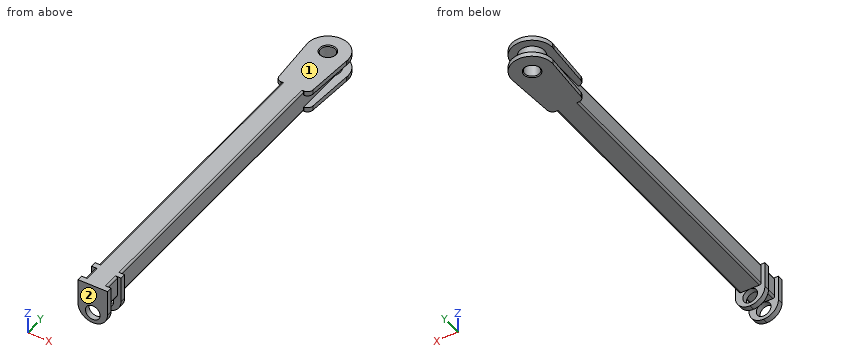
```python
from build123d import *

# Parameters (mm, degrees)
F0_W      = 120
F0_H      = 120
F0_W_2    = 100
F0_H_2    = 100
F1_DEPTH  = 1000
F2_R      = 67.5
F3_DEPTH  = 120
F4_R      = 40
F5_DEPTH  = 120
F7_DEPTH  = 25
F9_DEPTH  = 25
F10_R     = 40
F11_DEPTH = 160
F12_W     = 30
F12_H     = 220
F13_DEPTH = 140
F14_W     = 30
F14_H     = 220
F15_DEPTH = 20
F16_W     = 30
F16_H     = 220
F17_DEPTH = 140
F18_W     = 30
F18_H     = 220
F19_DEPTH = 20
F20_R     = 40
F21_DEPTH = 145
F22_R     = 10
F23_R     = 79.99999
F24_R     = 30
F25_SIZE  = 5


# Not quite as in the source:
# - a fillet or chamfer is up to 0.001 mm smaller than in the source, because OpenCascade refuses the exact size


with BuildPart() as f1:
    # F0 (on Front) → F1 (new body, symmetric)
    with BuildSketch(Plane.XZ):
        Rectangle(F0_W, F0_H)
        Rectangle(F0_W_2, F0_H_2, mode=Mode.SUBTRACT)
    extrude(amount=F1_DEPTH, both=True)

    # F2 (on face) → F3 (join)
    with BuildSketch(Plane.XY.offset(60)):
        with Locations((0, 1000)):
            Circle(F2_R)
    extrude(amount=-F3_DEPTH)

    # F4 (on face) → F5 (cut)
    with BuildSketch(Plane.XY.offset(60)):
        with Locations((0, 1000)):
            Circle(F4_R)
    extrude(amount=-F5_DEPTH, mode=Mode.SUBTRACT)

    # F6 (on face) → F7 (join)
    with BuildSketch(Plane.XY.offset(60)):
        with BuildLine():
            Line((109.0265486726, 985.3982300885), (110, 1000))
            ThreePointArc((110, 1000), (0, 1110), (-110, 1000))
            Line((-110, 1000), (-109.0265486726, 985.3982300885))
            ThreePointArc((-109.0265486726, 985.3982300885), (0, 890), (109.0265486726, 985.3982300885))
        make_face()
        with BuildLine():
            ThreePointArc((109.0265486726, 985.3982300885), (109.7563673642, 992.6829088424), (110, 1000))
            Line((110, 1000), (109.0265486726, 985.3982300885))
        make_face()
        with BuildLine():
            Line((-109.0265486726, 985.3982300885), (-110, 1000))
            ThreePointArc((-110, 1000), (-109.7563673642, 992.6829088424), (-109.0265486726, 985.3982300885))
        make_face()
        with BuildLine():
            Line((90, 700), (109.0265486726, 985.3982300885))
            ThreePointArc((109.0265486726, 985.3982300885), (0, 890), (-109.0265486726, 985.3982300885))
            Line((-109.0265486726, 985.3982300885), (-90, 700))
            Line((-90, 700), (90, 700))
        make_face()
    extrude(amount=-F7_DEPTH)

    # F8 (on face) → F9 (join)
    with BuildSketch(Plane(origin=(0, 0, -60), x_dir=(1, 0, 0), z_dir=(0, 0, -1))):
        with BuildLine():
            Line((109.0265486726, -985.3982300885), (110, -1000))
            ThreePointArc((110, -1000), (109.7563673642, -992.6829088424), (109.0265486726, -985.3982300885))
        make_face()
        with BuildLine():
            ThreePointArc((-109.7502513746, -992.5917395282), (-3.706234531, -1109.9375451136), (110, -1000))
            Line((110, -1000), (109.0265486726, -985.3982300885))
            ThreePointArc((109.0265486726, -985.3982300885), (-3.6149109138, -890.0594141407), (-109.7502513746, -992.5917395282))
        make_face()
        with BuildLine():
            ThreePointArc((-109.7502513746, -992.5917395282), (-3.6149109138, -890.0594141407), (109.0265486726, -985.3982300885))
            Line((109.0265486726, -985.3982300885), (90, -700))
            Line((90, -700), (-90, -700))
            Line((-90, -700), (-109.7502513746, -992.5917395282))
        make_face()
    extrude(amount=-F9_DEPTH)

    # F10 (on face) → F11 (cut)
    with BuildSketch(Plane(origin=(0, 0, -60), x_dir=(1, 0, 0), z_dir=(0, 0, -1))):
        with Locations((0, -1000)):
            Circle(F10_R)
    extrude(amount=-F11_DEPTH, mode=Mode.SUBTRACT)

    # F12 (on face) → F13 (join)
    with BuildSketch(Plane.YZ.offset(60)):
        with Locations((-870, -50)):
            Rectangle(F12_W, F12_H)
    extrude(amount=-F13_DEPTH)

    # F14 (on face) → F15 (join)
    with BuildSketch(Plane.YZ.offset(60)):
        with Locations((-870, -50)):
            Rectangle(F14_W, F14_H)
    extrude(amount=F15_DEPTH)

    # F16 (on face) → F17 (join)
    with BuildSketch(Plane.YZ.offset(60)):
        with Locations((-985, -50)):
            Rectangle(F16_W, F16_H)
    extrude(amount=-F17_DEPTH)

    # F18 (on face) → F19 (join)
    with BuildSketch(Plane.YZ.offset(60)):
        with Locations((-985, -50)):
            Rectangle(F18_W, F18_H)
    extrude(amount=F19_DEPTH)

    # F20 (on face) → F21 (cut)
    with BuildSketch(Plane.XZ.offset(1000)):
        with Locations((0, -100)):
            Circle(F20_R)
    extrude(amount=-F21_DEPTH, mode=Mode.SUBTRACT)

    # F22
    f22_edges = [f1.edges().sort_by_distance(p)[0] for p in [
        (60, -77.5, 60),
        (60, -77.5, -60),
        (60, -927.5, -60),
        (60, -927.5, 60),
        (-60, -77.5, 60),
        (-60, -927.5, 60),
        (-60, -927.5, -60),
        (-60, -77.5, -60),
    ]]
    fillet(f22_edges, radius=F22_R)

    # F23 (radius 80 in the source; OpenCascade refuses exactly that, so slightly less here)
    f23_edges = [f1.edges().sort_by_distance(p)[0] for p in [
        (-80, -985, -160),
        (80, -985, -160),
        (80, -870, -160),
        (-80, -870, -160),
    ]]
    fillet(f23_edges, radius=F23_R)

    # F24
    f24_edges = [f1.edges().sort_by_distance(p)[0] for p in [
        (-90, 700, -47.5),
        (-90, 700, 47.5),
        (90, 700, -47.5),
        (90, 700, 47.5),
    ]]
    fillet(f24_edges, radius=F24_R)

    # F25
    f25_edges = [f1.edges().sort_by_distance(p)[0] for p in [
        (-40, 1000, 60),
        (-40, 1000, -60),
    ]]
    chamfer(f25_edges, length=F25_SIZE)


solid = f1.part
```
Part model, mm, in its own coordinate system. Face numbers are marked on the shaded views. Round coordinates to 2 decimals unless told otherwise and drop trailing zeros. Write each loop counter-clockwise with the first axis right and the second up, starting at its lowest first coordinate (ties: lowest second). Pieces come first, ordered by that corner, then holes. Notation, with made-up numbers: M 71,83.25 L 77,83.25 A12 ccw 77,89.25 Z; hole C -1.5,42 d4. An arc over 180 degrees is marked long. One line per question, with ' | ' between items.
(1) Probe line 1 along Y through (x, z) = (0, 19); line 2 along X through (y, z) = (1000, -3); line 3 along X through (y, z) = (-414.5, -26). List the from-to ranges inside material, lowest first.
Answer key:
line 1: y = -1000 to -970, -885 to -855, 932.5 to 960, 1040 to 1067.5 | line 2: x = -67.5 to -40, 40 to 67.5 | line 3: x = -60 to -50, 50 to 60
(2) Two-plate mould, pull along Y, no slides. Class the marked faces 1 and 2: released by +Y, released by -Y, zero draft, split by the parting line, or undercut.
Answer key:
face 1: zero draft | face 2: released by -Y
(3) Saw through at B-B on z = -100. Write the cut outline in (x, y), then the cut area to 3 significant figures.
Answer key:
outline: M -77.46,-1000 L -40,-1000 L -40,-970 L -77.46,-970 Z; M -77.46,-885 L -40,-885 L -40,-855 L -77.46,-855 Z; M 40,-1000 L 77.46,-1000 L 77.46,-970 L 40,-970 Z; M 40,-885 L 77.46,-885 L 77.46,-855 L 40,-855 Z | area: 4,500 mm^2
(4) Pin check, flat tips, straight feed: pin 1 (1 mm diameter, centred on x = 20.5, z = -62, fed in from +Y); pin 2 (1 mm diameter, centred on x = 52, y = 206.5, fed in from +Z); pin 3 (2 mm diameter, centred on y = -757.5, z = 15.5, fed in from -X). Stop position of each tip, or through.
Answer key:
pin 1: stops at y = -855 | pin 2: stops at z = 59.89 | pin 3: stops at x = -60
(5) Saw through at A-A on y = -68. Write the cut outline in (x, z).
Answer key:
outline: M -60,-50 A10 ccw -50,-60 L 50,-60 A10 ccw 60,-50 L 60,50 A10 ccw 50,60 L -50,60 A10 ccw -60,50 Z; hole M -50,-50 L 50,-50 L 50,50 L -50,50 Z
